The model under review builds one solid part; all positions refer to its coordinate system, in mm. Face numbers are marked on the shaded views. A direction names the side the tool comes from. Round coordinates to 2 decimals unless told otherwise and drop trailing zeros. Write each loop counter-clockwise with the first axis right and the second up, starting at its lowest first coordinate (ties: lowest second). Pieces come first, ordered by that corner, then holes. Notation, with made-up numbers: (88.5, 5.5) - (133.5, 5.5) arc R21 cw to (133.5, 31.5) - close; hole circle Ø8 at (60.25, 13.5). An arc over 180 degrees is marked (long way). Use one line per item in the form item = value.
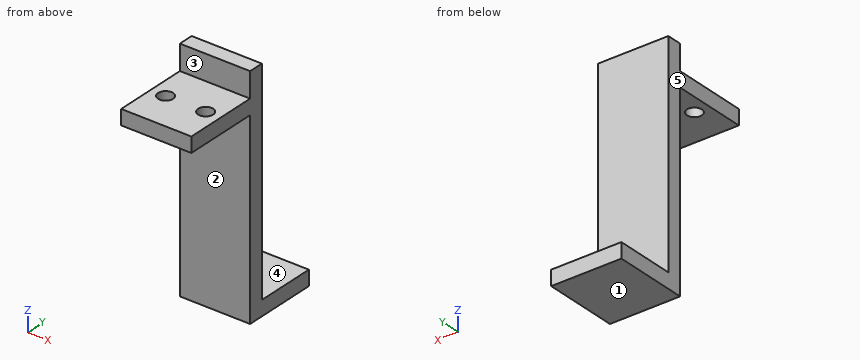
Autodesk Inventor part; units mm, degrees
ref_plane "YZ Plane" through (0, 0, 0) normal (1, 0, 0) x (0, 1, 0)
ref_plane "XZ Plane" through (0, 0, 0) normal (0, 1, 0) x (-1, 0, 0)
ref_plane "XY Plane" through (0, 0, 0) normal (0, 0, 1) x (1, 0, 0)
sketch "Sketch1" plane through (0, 0, 0) normal (0, 1, 0) x (-1, 0, 0)
  line L0 (0, 0) -> (14, 0)
  line L1 (14, 0) -> (14, -35)
  line L2 (14, -35) -> (0, -35)
  line L3 (0, -35) -> (0, 0)
  line L4 (14, -35) -> (0, -35)
  line L5 (0, -35) -> (0, -38)
  line L6 (0, -38) -> (14, -38)
  line L7 (14, -38) -> (14, -35)
  line L8 (14, 0) -> (0, 0)
  line L9 (0, 0) -> (0, 3)
  line L10 (0, 3) -> (14, 3)
  line L11 (14, 3) -> (14, 0)
  dimension "d0" = 14
  dimension "d1" = 35
  dimension "d2" = 3
  dimension "d3" = 3
extrude "Extrusion1" add sketch "Sketch1" along normal blind 3 contours L0 L1 L2 L3
extrude "Extrusion2" add sketch "Sketch1" along normal blind 15 contours L2 L7 L6 L5
extrude "Extrusion3" add sketch "Sketch1" along normal blind 3 and the other way blind 15 contours L9 L10 L11 L0
sketch "Sketch2" plane through (-14, 3, 3) normal (0, 0, 1) x (1, 0, 0)
  line L0 (0, 0) -> (14, 0)
  line L1 (14, 0) -> (14, -3)
  line L2 (14, -3) -> (0, -3)
  line L3 (0, -3) -> (0, 0)
  line L4 (0, 0) -> (14, 0)
extrude "Extrusion4" add sketch "Sketch2" along normal blind 5
sketch "Sketch3" plane through (-14, -15, 3) normal (0, 0, 1) x (1, 0, 0)
  line L0 (14, 0) -> (14, 15)
  line L1 (14, 15) -> (14, 11)
  line L2 (14, 0) -> (0, 0)
  line L3 (14, 0) -> (14, 4)
  line L4 (0, 0) -> (0, 15)
  line L5 (0, 0) -> (0, 4)
  line L6 (0, 15) -> (0, 11)
  line L7 (14, 7.5) -> (10, 7.5)
  line L8 (0, 7.5) -> (4, 7.5)
  line L9 (10, 7.5) -> (11, 7.5)
  circle A0 centre (11, 7.5) radius 1.5
  line L10 (4, 7.5) -> (1, 7.5)
  line L11 (4, 7.5) -> (3, 7.5)
  circle A1 centre (3, 7.5) radius 1.5
  dimension "d18" = 4
  dimension "d20" = 4
  dimension "d28" = 4
  dimension "d29" = 4
  dimension "d32" = 1
  dimension "d33" = 3
  dimension "d34" = 3
  dimension "d35" = 1
  dimension "d36" = 3
extrude "Extrusion5" cut sketch "Sketch3" against normal blind 5
properties part number "holder"
(1) Add section C-C on z = 1. Write out the cut boundary in (x, y).
Geometry results:
outline = (-14, -15) - (0, -15) - (0, 3) - (-14, 3) - close; hole circle Ø3 at (-11, -7.5); hole circle Ø3 at (-3, -7.5)
(2) Insertion check: P1, Ø8, axis at x = -8, y = -4.5, coming from the +Z side; P2, Ø6, axis at x = -5, z = -31, coming from the +Y side; P3, Ø4, axis at x = -5.5, z = -19.5, coming from the -Y side; P4, Ø1.8, axis at x = -3, y = -7.5, coming from the +Z side. Each pin has a flat end and moves straight along its axis. Give the tip position at first contact, or say it passes through.
Geometry results:
P1 = 3
P2 = 3
P3 = 0
P4 = through
(3) Add section D-D on x = -7.75. Write out the cut boundary in (y, z), then the cut area to 3 significant figures.
Geometry results:
outline = (-15, 0) - (0, 0) - (0, -38) - (15, -38) - (15, -35) - (3, -35) - (3, 8) - (0, 8) - (0, 3) - (-15, 3) - close
area = 219 mm2
(4) Add section B-B on x = -11. Write out the cut boundary in (y, z).
Geometry results:
outline = (-15, 0) - (-9, 0) - (-9, 3) - (-15, 3) - close; (-6, 0) - (0, 0) - (0, -38) - (15, -38) - (15, -35) - (3, -35) - (3, 8) - (0, 8) - (0, 3) - (-6, 3) - close
(5) To check wall thickness, follow L1, parallel to Y at x = -3, z = 0.6; L2, parallel to Y at x = -8.5, z = -26. State the ranges of each line that lie inside material, in increasing order.
Geometry results:
L1 = -15 to -9, -6 to 3
L2 = 0 to 3
(6) Machinability: for the marked faces 1, 2, 3, 4 and 5, which of the approach directions +Z, -Z, +X, -X, +Y, -Y give a long, thin tool a straight path to every point of the face, cutting with its end or side? Answer none if there is none.
Geometry results:
face_1 = -Z, +X, -X, +Y, -Y
face_2 = -Z, +X, -X, -Y
face_3 = +Z, +X, -X, -Y
face_4 = +Z, +X, -X, +Y
face_5 = +Z, -Z, -X, +Y, -Y
(7) Add section A-A on y = -7.5. Write out the cut boundary in (x, z).
Geometry results:
outline = (-14, 0) - (-12.5, 0) - (-12.5, 3) - (-14, 3) - close; (-9.5, 0) - (-4.5, 0) - (-4.5, 3) - (-9.5, 3) - close; (-1.5, 0) - (0, 0) - (0, 3) - (-1.5, 3) - close
